Read the model definition and answer for the solid it produces. Units are mm, in the model's axes. A direction names the side the tool comes from. Give positions to 0.01 mm unless a question says otherwise; leave off trailing zeros. Loops run counter-clockwise (first coordinate to the right, second up) from the corner with the lowest first, then second, coordinate; pieces in that order, holes last. Notation, with made-up numbers: (84.5, 5) - (123.5, 5) arc R21 ccw to (123.5, 31) - close; hole circle Ø9 at (54.25, 81.5). An arc over 180 degrees is marked (long way). Write each question's results on one line, items separated by ' | '. Start each with the question number.
Q1. Determine the mould class of faces 1 (the flat face through (41.275, 1, -8)), 2 (the cylindrical face through (-2.209, -23.183, -30.235)), 3 (the flat face through (38.1, -16, -16)), 4 (the flat face through (-3.175, 1, 8)) for opening direction X: +X half, -X half, draft (parallel to the pull), parting line (faces both ways), or undercut.
Q2. Given pin 1 (8 mm diameter, centred on x = 14, y = 11.5, fed in from +Z); pin 2 (1.5 mm diameter, centred on x = 14, y = 20, fed in from +Z); pin 3 (1.5 mm diameter, centred on x = 29, z = -11, fed in from -Y), each flat-ended and moving along its own axis, determine where each tip first touches the part or whether it passes through.
Q3. The part is cut by section B-B, the plane x = 9. Write down the section's boundary in (y, z), plus the area to 3 significant figures.
Q4. The part is cut by section A-A, the plane y = 0. Write down the section's boundary in (x, z) (3 decimals).
Q5. For faces 5 (the flat face through (0, -16, 16)), 6 (the flat face through (18.739, 0.673, 6.314)), determine the directions among +Z, -Z, +X, -X, +Y, -Y from which every point of the face is accessible in a straight line to the end or side of a thin tool.
Q6. Find the intervals of material crossed by line 1 (X direction, y = 33, z = -3) (3 decimals); line 2 (Z direction, x = 9, y = -3); line 3 (Y direction, x = 5, z = -7.5), in increasing order. Write a range as from..to.
```python
from build123d import *

# Parameters (mm, degrees)
SKETCH1_R           = 19.05
BOSS_EXTRUDE1_DEPTH = 38.1
SKETCH2_R           = 38.1
BOSS_EXTRUDE2_DEPTH = 3.175
SKETCH3_R           = 38.1
BOSS_EXTRUDE3_DEPTH = 3.175
SKETCH4_R           = 6.35
CUT_EXTRUDE1_DEPTH  = 45.45
FILLET1_R           = 1.27
CUT_EXTRUDE2_DEPTH  = 45.45


with BuildPart() as part:
    # Sketch1 → Boss-Extrude1 (new body)
    with BuildSketch(Plane(origin=(0, 0, 0), x_dir=(0, 0, -1), z_dir=(1, 0, 0))):
        Circle(SKETCH1_R)
    extrude(amount=BOSS_EXTRUDE1_DEPTH)

    # Sketch2 → Boss-Extrude2 (add)
    with BuildSketch(Plane.ZY):
        Circle(SKETCH2_R)
    extrude(amount=BOSS_EXTRUDE2_DEPTH)

    # Sketch3 → Boss-Extrude3 (add)
    with BuildSketch(Plane(origin=(38.1, 0, 0), x_dir=(0, 0, -1), z_dir=(1, 0, 0))):
        Circle(SKETCH3_R)
    extrude(amount=BOSS_EXTRUDE3_DEPTH)

    # Sketch4 → Cut-Extrude1 (cut, through all)
    with BuildSketch(Plane.ZY.offset(3.175)):
        Circle(SKETCH4_R)
    extrude(amount=-CUT_EXTRUDE1_DEPTH, mode=Mode.SUBTRACT)

    # Fillet1
    fillet1_edges = [part.edges().sort_by_distance(p)[0] for p in [
        (0, 0, -38.1),
        (38.1, 0, 38.1),
    ]]
    fillet(fillet1_edges, radius=FILLET1_R)

    # Sketch5 → Cut-Extrude2 (cut, through all)
    with BuildSketch(Plane.ZY.offset(3.175)):
        Polygon((-5.890350999, -4.366588879), (0.836401397, -7.284488042), (6.726752397, -2.917899163), (5.890350999, 4.366588879), (-0.836401397, 7.284488042), (-6.726752397, 2.917899163), align=None)
    extrude(amount=-CUT_EXTRUDE2_DEPTH, mode=Mode.SUBTRACT)


solid = part.part
```
Check sheet entries:
1) face 1: +X half | face 2: draft | face 3: undercut | face 4: -X half
2) pin 1: stops at z = 17.51 | pin 2: passes through | pin 3: stops at y = -16.06
3) outline: circle Ø38.1 at (0, 0); hole (-7.28, 0.84) - (-4.37, -5.89) - (2.92, -6.73) - (7.28, -0.84) - (4.37, 5.89) - (-2.92, 6.73) - close | area: 1,000 mm^2
4) outline: (-3.175, -38.1) - (-1.27, -38.1) arc R1.27 ccw to (0, -36.83) - (0, -19.05) - (38.1, -19.05) - (38.1, -36.83) arc R1.27 ccw to (39.37, -38.1) - (41.275, -38.1) - (41.275, -6.392) - (-3.175, -6.392) - close; (-3.175, 6.392) - (41.275, 6.392) - (41.275, 38.1) - (39.37, 38.1) arc R1.27 ccw to (38.1, 36.83) - (38.1, 19.05) - (0, 19.05) - (0, 36.83) arc R1.27 ccw to (-1.27, 38.1) - (-3.175, 38.1) - close
5) face 5: none | face 6: +X, -X
6) line 1: x = -3.175..0, 38.1..41.275 | line 2: z = -18.81..-6.05, 6.62..18.81 | line 3: y = -17.51..17.51
